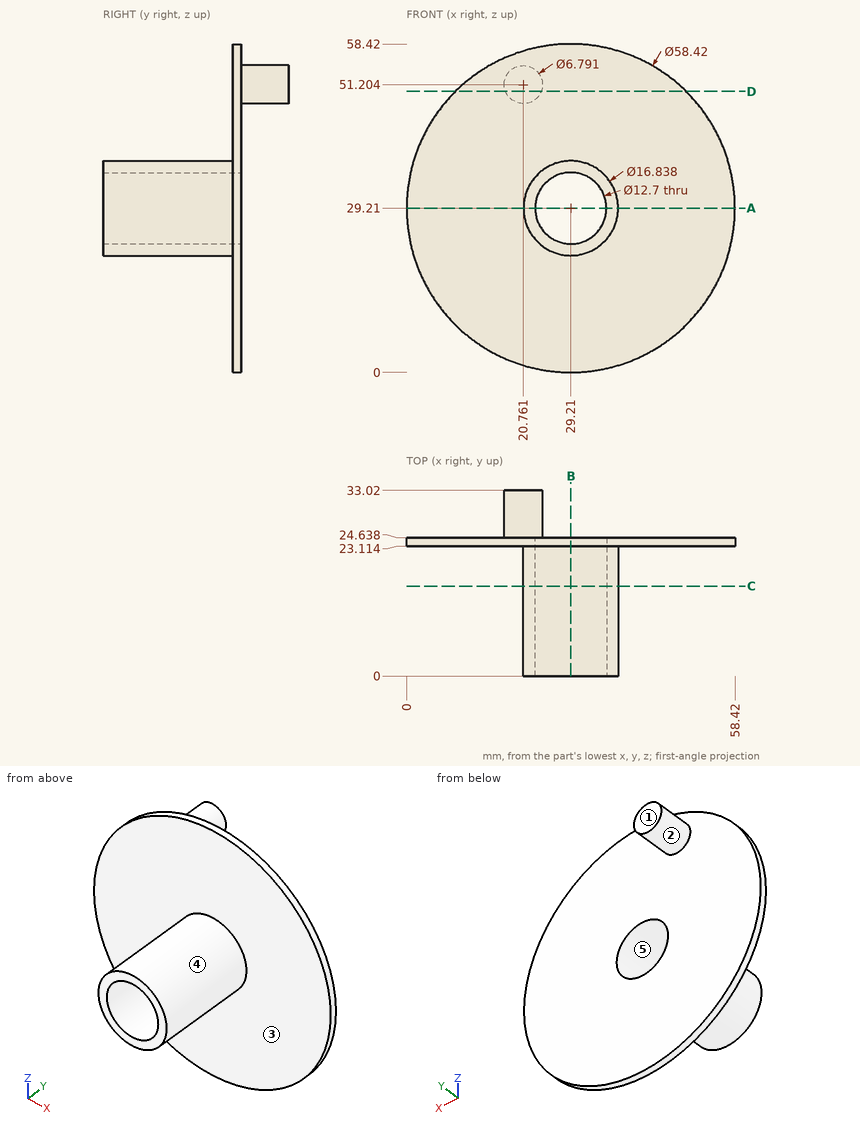
Drawing for the job (mm, zero at the part's lowest x, y, z). A direction names the side the tool comes from. Round coordinates to 2 decimals unless told otherwise and drop trailing zeros. Write each loop counter-clockwise with the first axis right and the second up, starting at its lowest first coordinate (ties: lowest second). Pieces come first, ordered by that corner, then holes. Notation, with made-up numbers: M 34.25,-16.5 L 44.25,-16.5 A15 cw 44.25,-11.5 Z; hole C -27,55 d8. An arc over 180 degrees is marked long. Answer in a Markdown table with one row per item.
1. Saw through at B-B (x = 29.21). List the corners of the cut face in (y, z).
Geometry check:
| item | result |
|---|---|
| outline | M 0,20.79 L 23.11,20.79 L 23.11,0 L 24.64,0 L 24.64,22.86 L 0,22.86 Z; M 0,35.56 L 24.64,35.56 L 24.64,58.42 L 23.11,58.42 L 23.11,37.63 L 0,37.63 Z |
2. Saw through at A-A (z = 29.21). List the corners of the cut face in (x, y), and give its area (3 significant figures).
Geometry check:
| item | result |
|---|---|
| outline | M 0,23.11 L 20.79,23.11 L 20.79,0 L 22.86,0 L 22.86,24.64 L 0,24.64 Z; M 35.56,0 L 37.63,0 L 37.63,23.11 L 58.42,23.11 L 58.42,24.64 L 35.56,24.64 Z |
| area | 165 mm2 |
3. Saw through at D-D (z = 50). List the corners of the cut face in (x, y) (1 decimal), and give its area (3 significant figures).
Geometry check:
| item | result |
|---|---|
| outline | M 8.7,23.1 L 49.7,23.1 L 49.7,24.6 L 23.9,24.6 L 23.9,33 L 17.6,33 L 17.6,24.6 L 8.7,24.6 Z |
| area | 116 mm2 |
4. Saw through at C-C (y = 16). List the corners of the cut face in (x, z).
Geometry check:
| item | result |
|---|---|
| outline | C 29.21,29.21 d16.84; hole C 29.21,29.21 d12.7 |
5. Probe L1, parallel to X at y = 18, z = 29; L2, parallel to Z at x = 31, y = 11 (1 decimal). List the from-to ranges inside material, lowest first. Write a range as [from, to].
Geometry check:
| item | result |
|---|---|
| L1 | [20.79, 22.86], [35.56, 37.63] |
| L2 | [21, 23.1], [35.3, 37.4] |
6. Flat gauge pins, fed straight in: P1, Ø8, axis at x = 9.5, z = 28, coming from the -Y side; P2, Ø8, axis at y = 20.5, z = 10.5, coming from the +X side; P3, Ø5, axis at y = 23.5, z = 13.5, coming from the +X side. Where does each tip first touch, or does it go through?
Geometry check:
| item | result |
|---|---|
| P1 | y = 23.11 |
| P2 | x = 53.85 |
| P3 | x = 55.26 |
7. Which spindle directions (+Z, -Z, +X, -X, +Y, -Y) get a long thin tool onto all of the face, cutting with end or side? Do the marked faces 1 and 2. Say none if no direction does.
Geometry check:
| item | result |
|---|---|
| face 1 | +Z, -Z, +X, -X, +Y |
| face 2 | +Y |
8. Mould opens along X. For the marked faces 3, 4 and 5 say: +X half, -X half, draft (parallel to the pull), parting line (faces both ways), or undercut.
Geometry check:
| item | result |
|---|---|
| face 3 | draft |
| face 4 | parting line |
| face 5 | undercut |
